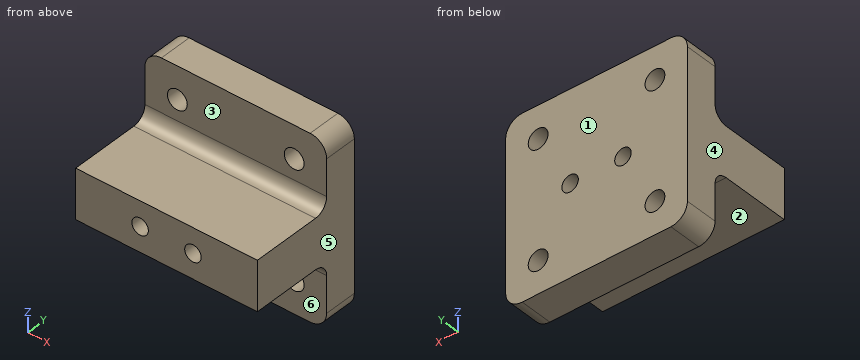
```python
from build123d import *

# Parameters (mm, degrees)
F0_W          = 55
F0_H          = 55
F0_R          = 3
F1_DEPTH      = 10
F2_R          = 5
F3_W          = 25
F3_H          = 15
F4_DEPTH      = 55
F5_R          = 2.5
F6_DEPTH      = 10.001
F6_DEPTH_BACK = 25.001
F7_R          = 4


with BuildPart() as f1:
    # F0 (on Front) → F1 (new body)
    with BuildSketch(Plane.XZ):
        Rectangle(F0_W, F0_H)
        with Locations((-17.6776695297, -17.6776695297)):
            Circle(F0_R, mode=Mode.SUBTRACT)
        with Locations((17.6776695297, -17.6776695297)):
            Circle(F0_R, mode=Mode.SUBTRACT)
        with Locations((-17.6776695297, 17.6776695297)):
            Circle(F0_R, mode=Mode.SUBTRACT)
        with Locations((17.6776695297, 17.6776695297)):
            Circle(F0_R, mode=Mode.SUBTRACT)
    extrude(amount=F1_DEPTH)

    # F2
    f2_edges = [f1.edges().sort_by_distance(p)[0] for p in [
        (-27.5, -5, 27.5),
        (-27.5, -5, -27.5),
        (27.5, -5, 27.5),
        (27.5, -5, -27.5),
    ]]
    fillet(f2_edges, radius=F2_R)

    # F3 (on face) → F4 (join)
    with BuildSketch(Plane.YZ.offset(27.5)):
        with Locations((-22.5, 0)):
            Rectangle(F3_W, F3_H)
    extrude(amount=-F4_DEPTH)

    # F5 (on face) → F6 (cut, two sides)
    with BuildSketch(Plane.XZ.offset(10)) as f6_sk:
        with Locations((8, 0)):
            Circle(F5_R)
        with Locations((-8, 0)):
            Circle(F5_R)
    extrude(amount=-F6_DEPTH, mode=Mode.SUBTRACT)
    extrude(f6_sk.sketch, amount=F6_DEPTH_BACK, mode=Mode.SUBTRACT)

    # F7
    f7_edges = [f1.edges().sort_by_distance(p)[0] for p in [
        (0, -10, -7.5),
        (0, -10, 7.5),
    ]]
    fillet(f7_edges, radius=F7_R)


solid = f1.part
```
For this review, take the finished solid that the model builds, in its own axes (mm). Face numbers are marked on the shaded views. A direction names the side the tool comes from. Coordinates: 2 decimals unless noted, no trailing zeros. Write each loop counter-clockwise with the first axis right and the second up, starting at its lowest first coordinate (ties: lowest second). Pieces come first, ordered by that corner, then holes. Notation, with made-up numbers: (61.25, 38) -> (71.25, 38) arc R13 cw to (71.25, 56) -> close; hole circle Ø3 at (88, 53). An arc over 180 degrees is marked (long way). Put each result on its own line as item: value.
Q1. Take a section at B-B, the plane x = -8. State the section outline as (y, z) points, then the cut area to 3 significant figures.
From the geometry:
outline: (-35, -7.5) -> (-14, -7.5) arc R4 cw to (-10, -11.5) -> (-10, -27.5) -> (0, -27.5) -> (0, -2.5) -> (-35, -2.5) -> close; (-35, 2.5) -> (0, 2.5) -> (0, 27.5) -> (-10, 27.5) -> (-10, 11.5) arc R4 cw to (-14, 7.5) -> (-35, 7.5) -> close
area: 757 mm2
Q2. Take a section at C-C, the plane y = -28.5. State the section outline as (x, z) points.
From the geometry:
outline: (-27.5, -7.5) -> (27.5, -7.5) -> (27.5, 7.5) -> (-27.5, 7.5) -> close; hole circle Ø5 at (-8, 0); hole circle Ø5 at (8, 0)
Q3. Take a section at D-D, the plane x = 18.5. State the section outline as (y, z) points.
From the geometry:
outline: (-35, -7.5) -> (-14, -7.5) arc R4 cw to (-10, -11.5) -> (-10, -14.79) -> (0, -14.79) -> (0, 14.79) -> (-10, 14.79) -> (-10, 11.5) arc R4 cw to (-14, 7.5) -> (-35, 7.5) -> close; (-10, -27.5) -> (0, -27.5) -> (0, -20.56) -> (-10, -20.56) -> close; (-10, 20.56) -> (0, 20.56) -> (0, 27.5) -> (-10, 27.5) -> close
Q4. The part is to be moulded in two halves that separate along X. For the marked faces 4, 5 and 6, say which applies: +X half, -X half, draft (parallel to the pull), parting line (faces both ways), or undercut.
From the geometry:
face 4: -X half
face 5: +X half
face 6: draft
Q5. Clearance check with flat-ended pins moving along their axes: pin 1 Ø7 at (x, z) = (-17.68, 17.68) entering from -Y; pin 2 Ø1 at (x, y) = (5, -15.5) entering from +Z; pin 3 Ø10.5 at (x, y) = (-8, -23.5) entering from -Z. State where each tip first meets the part, or that it passes through.
From the geometry:
pin 1: stops at y = -10
pin 2: stops at z = 7.5
pin 3: stops at z = -7.5
Q6. Tool access review of the marked faces 1, 2 and 3: name each direction out of +Z, -Z, +X, -X, +Y, -Y from which nothing blocks a thin tool from reaching the whole face with its end or side.
From the geometry:
face 1: +Z, -Z, +X, -X, +Y
face 2: -Z, +X, -X, -Y
face 3: +Z, +X, -X, -Y
Q7. Wall thickness on L1, parallel to X at y = -17, z = 2; L2, parallel to X at y = -3.5, z = 19; L3, parallel to Z at x = -17, y = -7.5: over which ranges is each line inside the solid? List them lowest first.
From the geometry:
L1: x = -27.5 to -9.5, -6.5 to 6.5, 9.5 to 27.5
L2: x = -27.5 to -20.37, -14.98 to 14.98, 20.37 to 27.5
L3: z = -27.5 to -20.6, -14.76 to 14.76, 20.6 to 27.5
Q8. Take a section at A-A, the plane z = 0. State the section outline as (x, y) points, then the cut area to 4 significant figures.
From the geometry:
outline: (-27.5, -35) -> (-10.5, -35) -> (-10.5, 0) -> (-27.5, 0) -> close; (-5.5, -35) -> (5.5, -35) -> (5.5, 0) -> (-5.5, 0) -> close; (10.5, -35) -> (27.5, -35) -> (27.5, 0) -> (10.5, 0) -> close
area: 1,575 mm2
